```python
from build123d import *

# Parameters (mm, degrees)
SKETCH1_R           = 2
BOSS_EXTRUDE2_DEPTH = 2
BOSS_EXTRUDE3_START = -22
BOSS_EXTRUDE3_DEPTH = 22
FILLET1_R           = 15
FILLET2_R           = 3
SKETCH3_R           = 2
CUT_EXTRUDE1_DEPTH  = 21


with BuildPart() as part:
    # Sketch1 → Boss-Extrude2 (new body)
    # profile 1 of 5: a face of its own
    with BuildSketch(Plane.XY):
        with BuildLine():
            Line((-22.5, 19.5), (-22.5, -8))
            Line((-22.5, -8), (-11.489125293, -8))
            ThreePointArc((-11.489125293, -8), (-4.192388692, 13.357540082), (14, 0))
            ThreePointArc((14, 0), (13.357540082, -4.192388692), (11.489125293, -8))
            Line((11.489125293, -8), (22.5, -8))
            Line((22.5, -8), (22.5, 19.5))
            Line((22.5, 19.5), (-22.5, 19.5))
        make_face()
        with Locations((-17.5, 0)):
            Circle(SKETCH1_R, mode=Mode.SUBTRACT)
        with Locations((17.5, 0)):
            Circle(SKETCH1_R, mode=Mode.SUBTRACT)
    # profile 2 of 5: a face of its own
    with BuildSketch(Plane.XY):
        with BuildLine():
            ThreePointArc((14, 0), (-4.192388692, 13.357540082), (-11.489125293, -8))
            Line((-11.489125293, -8), (-4.75, -8))
            ThreePointArc((-4.75, -8), (0, -3.25), (4.75, -8))
            Line((4.75, -8), (11.489125293, -8))
            ThreePointArc((11.489125293, -8), (13.357540082, -4.192388692), (14, 0))
        make_face()
    # profile 3 of 5: a face of its own
    with BuildSketch(Plane.XY):
        with BuildLine():
            Line((-4.75, -8), (-11.489125293, -8))
            ThreePointArc((-11.489125293, -8), (0, -14), (11.489125293, -8))
            Line((11.489125293, -8), (4.75, -8))
            ThreePointArc((4.75, -8), (0, -12.75), (-4.75, -8))
        make_face()
    # profile 4 of 5: a face of its own
    with BuildSketch(Plane.XY):
        with BuildLine():
            ThreePointArc((14, 0), (-4.192388692, 13.357540082), (-11.489125293, -8))
            Line((-11.489125293, -8), (-4.75, -8))
            ThreePointArc((-4.75, -8), (0, -3.25), (4.75, -8))
            Line((4.75, -8), (11.489125293, -8))
            ThreePointArc((11.489125293, -8), (13.357540082, -4.192388692), (14, 0))
        make_face()
    # profile 5 of 5: a face of its own
    with BuildSketch(Plane.XY):
        with BuildLine():
            Line((-4.75, -8), (-11.489125293, -8))
            ThreePointArc((-11.489125293, -8), (0, -14), (11.489125293, -8))
            Line((11.489125293, -8), (4.75, -8))
            ThreePointArc((4.75, -8), (0, -12.75), (-4.75, -8))
        make_face()
    extrude(amount=BOSS_EXTRUDE2_DEPTH)

    # Sketch2 → Boss-Extrude3 (add)
    with BuildSketch(Plane.XY.offset(2).offset(BOSS_EXTRUDE3_START)):
        with BuildLine():
            Line((-22.5, -8), (-22.5, -10))
            Line((-22.5, -10), (-12.489995997, -10))
            ThreePointArc((-12.489995997, -10), (0, -16), (12.489995997, -10))
            Line((12.489995997, -10), (22.5, -10))
            Line((22.5, -10), (22.5, -8))
            Line((22.5, -8), (11.489125293, -8))
            ThreePointArc((11.489125293, -8), (0, -14), (-11.489125293, -8))
            Line((-11.489125293, -8), (-22.5, -8))
        make_face()
    extrude(amount=BOSS_EXTRUDE3_DEPTH)

    # Fillet1
    fillet1_edges = [part.edges().sort_by_distance(p)[0] for p in [
        (-22.5, 19.5, 1),
        (22.5, 19.5, 1),
    ]]
    fillet(fillet1_edges, radius=FILLET1_R)

    # Fillet2
    fillet2_edges = [part.edges().sort_by_distance(p)[0] for p in [
        (-16.994562647, -8, 0),
        (16.994562647, -8, 0),
    ]]
    fillet(fillet2_edges, radius=FILLET2_R)

    # Sketch3 → Cut-Extrude1 (cut)
    with BuildSketch(Plane(origin=(0, -8, 0), x_dir=(1, 0, 0), z_dir=(0, 1, 0))):
        with Locations(Location((-16.994562647, 6, 0), (0, 0, 270))):
            Circle(SKETCH3_R)
        with Locations(Location((-16.994562647, 17, 0), (0, 0, 270))):
            Circle(SKETCH3_R)
        with Locations(Location((16.994562647, 17, 0), (0, 0, 270))):
            Circle(SKETCH3_R)
        with Locations(Location((16.994562647, 6, 0), (0, 0, 270))):
            Circle(SKETCH3_R)
    extrude(amount=-CUT_EXTRUDE1_DEPTH, mode=Mode.SUBTRACT)


solid = part.part
```
Input: part model. Units: mm. Frame: model coordinates. A direction names the side the tool comes from. Give positions to 0.01 mm unless a question says otherwise; leave off trailing zeros. Order: outer loops, then holes, each group sorted by start corner. A loop starts at its lowest first (then second) coordinate and runs counter-clockwise, first axis right, second up. Notation, with made-up numbers: (-37.5, -14.5) -> (-21.5, -14.5) arc R16 cw to (-21.5, -4.5) -> close; hole circle Ø11 at (-2, 24.5). An arc over 180 degrees is marked (long way). Write each question's results on one line, items separated by ' | '. Start each with the question number.
Item 1: Cut plane C-C on z = -3.5. Return the cut outline in (x, y), then the cut area to 3 significant figures.
Item 2: Mould query, pull axis Z, two halves, no side actions, for faces 1 (the flat face through (17, -10, -9)), 2 (the cylindrical face through (-16.92, -7.1, -0.86)), 3 (the cylindrical face through (-18.947, -8.986, -17.434)). Classes: pulls with the +Z half, pulls with the -Z half, needs draft (parallel to the pull), parting line crosses it, or undercut.
Item 3: Set-up query: faces 4 (the cylindrical face through (-1.03, -3.363, 0.986)), 5 (the flat face through (-17, -8, -12)), 6 (the cylindrical face through (0, -14, -10)). Return all of +Z, -Z, +X, -X, +Y, -Y with unobstructed straight access to the full face (end or side cutting, diameter ignored); none if empty.
Item 4: Line query: line 1 (X direction, y = -9, z = -17); line 2 (X direction, y = -9.3, z = -17); line 3 (Y direction, x = 0, z = 1.2). Output: solid intervals per line, ascending.
Item 5: Cut plane A-A on x = 0. Return the cut outline in (y, z), then the cut area to 3 significant figures.
Item 6: Contact query for flat-ended pins moving along their axis: P1, Ø3.5, axis at x = 19.5, z = -10.5, coming from the +Y side; P2, Ø1, axis at x = 9.5, z = -14, coming from the -Y side; P3, Ø11, axis at x = -16, z = -11, coming from the -Y side; P4, Ø5.5, axis at x = 0, y = -8, coming from the +Z side. Output: stop coordinate, or through.
Item 7: Cut plane B-B on y = 0. Return the cut outline in (x, z), then the cut area to 3 significant figures.
Item 8: Cut plane D-D on z = -17. Return the cut outline in (x, y).
Established:
1) outline: (-22.5, -10) -> (-12.49, -10) arc R16 ccw to (12.49, -10) -> (22.5, -10) -> (22.5, -8) -> (11.49, -8) arc R14 cw to (-11.49, -8) -> (-22.5, -8) -> close | area: 97.6 mm^2
2) face 1: needs draft | face 2: pulls with the -Z half | face 3: undercut
3) face 4: +Z, -Z | face 5: -Z, +X, -X, +Y | face 6: -Z, +Y
4) line 1: -22.5 to -18.99, -14.99 to -10.72, 10.72 to 14.99, 18.99 to 22.5 | line 2: -22.5 to -18.99, -14.99 to -10.46, 10.46 to 14.99, 18.99 to 22.5 | line 3: -16 to -12.75, -3.25 to 19.5
5) outline: (-16, -20) -> (-14, -20) -> (-14, 0) -> (-12.75, 0) -> (-12.75, 2) -> (-16, 2) -> close; (-3.25, 0) -> (19.5, 0) -> (19.5, 2) -> (-3.25, 2) -> close | area: 92.0 mm^2
6) P1: y = -8 | P2: y = -13.23 | P3: y = -12.07 | P4: through
7) outline: (-22.5, 0) -> (-19.5, 0) -> (-19.5, 2) -> (-22.5, 2) -> close; (-15.5, 0) -> (15.5, 0) -> (15.5, 2) -> (-15.5, 2) -> close; (19.5, 0) -> (22.5, 0) -> (22.5, 2) -> (19.5, 2) -> close | area: 74.0 mm^2
8) outline: (-22.5, -10) -> (-18.99, -10) -> (-18.99, -8) -> (-22.5, -8) -> close; (-14.99, -10) -> (-12.49, -10) arc R16 ccw to (12.49, -10) -> (14.99, -10) -> (14.99, -8) -> (11.49, -8) arc R14 cw to (-11.49, -8) -> (-14.99, -8) -> close; (18.99, -10) -> (22.5, -10) -> (22.5, -8) -> (18.99, -8) -> close
